Source: CAD feature listing. Evaluate the final solid. Frame: model axes, mm. A direction names the side the tool comes from. Coordinates: 2 decimals unless noted, no trailing zeros. Write each loop counter-clockwise with the first axis right and the second up, starting at its lowest first coordinate (ties: lowest second). Pieces come first, ordered by that corner, then holes. Notation, with made-up numbers: (53.5, -11.75) - (87.5, -11.75) arc R16 ccw to (87.5, 16.25) - close; hole circle Ø6 at (82.25, -23.75). An arc over 180 degrees is marked (long way). One line per question, with ' | ' between items. Start each with the question number.
Q1. Access query for faces 5 (the face through (-116, 4, 58)), 6 (the face through (-121, 3.5, -71)), 7 (the face through (116, 4, 58)), 8 (the face through (104.9, 3.8, -65)). Directions: +Z, -Z, +X, -X, +Y, -Y. A direction counts if a zero-diameter tool reaches every point of the face in a straight line with its end or side. Return the directions, or none.
Q2. Contact query for flat-ended pins moving along their axis: P1, Ø5, axis at x = 60.16, z = -71, coming from the +Y side; P2, Ø1, axis at y = 4.5, z = 50.5, coming from the +X side; P3, Ø1.7, axis at x = -120.5, z = -70, coming from the -Y side; P4, Ø3, axis at x = -122.5, z = 5, coming from the +Y side. Output: stop coordinate, or through.
Q3. Cut plane A-A, the plane z = -3. Return loops of the section in (x, y).
Q4. Line query: line 1 (X direction, y = 3.15, z = 60); line 2 (Z direction, x = 3.5, y = 3.6); line 3 (X direction, y = 3.7, z = -16). Output: solid intervals per line, ascending.
Q5. Draft query along Z for faces 1 (the face through (1, 5, -1)), 2 (the face through (119, 3.5, 69)), 3 (the face through (-121, 3.5, 69)), 4 (the face through (2, 2, 75)). Return one class per face: +Z half, -Z half, draft (parallel to the pull), parting line (faces both ways), or undercut.
```python
from build123d import *

# Parameters (mm, degrees)
EXTRUDE_1_DEPTH     = 5
CUT_EXTRUDE_1_DEPTH = 1.5
CUT_EXTRUDE_2_DEPTH = 2.5
SKETCH_4_R          = 1.25
CUT_EXTRUDE_3_DEPTH = 5
SKETCH_5_R          = 2.85
CUT_EXTRUDE_4_DEPTH = 3.5
SKETCH_6_R          = 1.25
CUT_EXTRUDE_5_DEPTH = 5
SKETCH_7_R          = 2.85
CUT_EXTRUDE_6_DEPTH = 3.5


with BuildPart() as part:
    # 草图1 → 凸台-拉伸1 (new body)
    with BuildSketch(Plane(origin=(0, 0, 0), x_dir=(1, 0, 0), z_dir=(0, 1, 0))):
        with BuildLine():
            Line((-120, 75), (120, 75))
            ThreePointArc((120, 75), (123.535533906, 73.535533906), (125, 70))
            Line((125, 70), (125, -70))
            ThreePointArc((125, -70), (123.535533906, -73.535533906), (120, -75))
            Line((120, -75), (-120, -75))
            ThreePointArc((-120, -75), (-123.535533906, -73.535533906), (-125, -70))
            Line((-125, -70), (-125, 70))
            ThreePointArc((-125, 70), (-123.535533906, 73.535533906), (-120, 75))
        make_face()
    extrude(amount=EXTRUDE_1_DEPTH)

    # 草图2 → 切除-拉伸1 (cut)
    with BuildSketch(Plane(origin=(0, 5, 0), x_dir=(1, 0, 0), z_dir=(0, 1, 0))):
        with BuildLine():
            Line((-125, 60), (-120, 60))
            ThreePointArc((-120, 60), (-116.464466094, 58.535533906), (-115, 55))
            Line((-115, 55), (-115, -55))
            ThreePointArc((-115, -55), (-116.464466094, -58.535533906), (-120, -60))
            Line((-120, -60), (-125, -60))
            Line((-125, -60), (-125, 60))
        make_face()
        with BuildLine():
            Line((115, 55), (115, -55))
            ThreePointArc((115, -55), (116.464466094, -58.535533906), (120, -60))
            Line((120, -60), (125, -60))
            Line((125, -60), (125, 60))
            Line((125, 60), (120, 60))
            ThreePointArc((120, 60), (116.464466094, 58.535533906), (115, 55))
        make_face()
    extrude(amount=-CUT_EXTRUDE_1_DEPTH, mode=Mode.SUBTRACT)

    # 草图3 → 切除-拉伸2 (cut)
    with BuildSketch(Plane(origin=(0, 5, 0), x_dir=(1, 0, 0), z_dir=(0, 1, 0))):
        with BuildLine():
            Line((-100, 67), (100, 67))
            ThreePointArc((100, 67), (104.949747468, 64.949747468), (107, 60))
            Line((107, 60), (107, -60))
            ThreePointArc((107, -60), (104.949747468, -64.949747468), (100, -67))
            Line((100, -67), (-100, -67))
            ThreePointArc((-100, -67), (-104.949747468, -64.949747468), (-107, -60))
            Line((-107, -60), (-107, 60))
            ThreePointArc((-107, 60), (-104.949747468, 64.949747468), (-100, 67))
        make_face()
        with BuildLine():
            Line((-100, 65), (100, 65))
            ThreePointArc((100, 65), (103.535533906, 63.535533906), (105, 60))
            Line((105, 60), (105, -60))
            ThreePointArc((105, -60), (103.535533906, -63.535533906), (100, -65))
            Line((100, -65), (-100, -65))
            ThreePointArc((-100, -65), (-103.535533906, -63.535533906), (-105, -60))
            Line((-105, -60), (-105, 60))
            ThreePointArc((-105, 60), (-103.535533906, 63.535533906), (-100, 65))
        make_face(mode=Mode.SUBTRACT)
    extrude(amount=-CUT_EXTRUDE_2_DEPTH, mode=Mode.SUBTRACT)

    # 草图4 → 切除-拉伸3 (cut)
    with BuildSketch(Plane.XZ):
        with Locations(Location((-120, 70, 0), (0, 0, 270))):
            Circle(SKETCH_4_R)
        with Locations(Location((-120, -70, 0), (0, 0, 270))):
            Circle(SKETCH_4_R)
        with Locations(Location((120, -70, 0), (0, 0, 270))):
            Circle(SKETCH_4_R)
        with Locations(Location((120, 70, 0), (0, 0, 270))):
            Circle(SKETCH_4_R)
    extrude(amount=-CUT_EXTRUDE_3_DEPTH, mode=Mode.SUBTRACT)

    # 草图5 → 切除-拉伸4 (cut)
    with BuildSketch(Plane.XZ):
        with Locations(Location((-120, 70, 0), (0, 0, 270))):
            Circle(SKETCH_5_R)
        with Locations(Location((-120, -70, 0), (0, 0, 270))):
            Circle(SKETCH_5_R)
        with Locations(Location((120, -70, 0), (0, 0, 270))):
            Circle(SKETCH_5_R)
        with Locations(Location((120, 70, 0), (0, 0, 270))):
            Circle(SKETCH_5_R)
    extrude(amount=-CUT_EXTRUDE_4_DEPTH, mode=Mode.SUBTRACT)

    # 草图6 → 切除-拉伸5 (cut)
    with BuildSketch(Plane(origin=(0, 5, 0), x_dir=(1, 0, 0), z_dir=(0, 1, 0))):
        with Locations(Location((0, 71, 0), (0, 0, 270))):
            Circle(SKETCH_6_R)
        with Locations(Location((-60.164669271, 71, 0), (0, 0, 270))):
            Circle(SKETCH_6_R)
        with Locations(Location((60.164669271, 71, 0), (0, 0, 90))):
            Circle(SKETCH_6_R)
        with Locations(Location((60.164669271, -71, 0), (0, 0, 270))):
            Circle(SKETCH_6_R)
        with Locations(Location((-60.164669271, -71, 0), (0, 0, 90))):
            Circle(SKETCH_6_R)
        with Locations(Location((0, -71, 0), (0, 0, 90))):
            Circle(SKETCH_6_R)
    extrude(amount=-CUT_EXTRUDE_5_DEPTH, mode=Mode.SUBTRACT)

    # 草图7 → 切除-拉伸6 (cut)
    with BuildSketch(Plane.XZ):
        with Locations(Location((-60.164669271, 71, 0), (0, 0, 270))):
            Circle(SKETCH_7_R)
        with Locations(Location((0, 71, 0), (0, 0, 270))):
            Circle(SKETCH_7_R)
        with Locations(Location((60.164669271, 71, 0), (0, 0, 270))):
            Circle(SKETCH_7_R)
        with Locations(Location((60.164669271, -71, 0), (0, 0, 90))):
            Circle(SKETCH_7_R)
        with Locations(Location((0, -71, 0), (0, 0, 90))):
            Circle(SKETCH_7_R)
        with Locations(Location((-60.164669271, -71, 0), (0, 0, 90))):
            Circle(SKETCH_7_R)
    extrude(amount=-CUT_EXTRUDE_6_DEPTH, mode=Mode.SUBTRACT)


solid = part.part
```
Reply:
1) face 5: -X, +Y | face 6: -Y | face 7: +X, +Y | face 8: +Y
2) P1: stops at y = 5 | P2: stops at x = 115 | P3: stops at y = 3.5 | P4: stops at y = 3.5
3) outline: (-125, 0) - (125, 0) - (125, 3.5) - (115, 3.5) - (115, 5) - (107, 5) - (107, 2.5) - (105, 2.5) - (105, 5) - (-105, 5) - (-105, 2.5) - (-107, 2.5) - (-107, 5) - (-115, 5) - (-115, 3.5) - (-125, 3.5) - close
4) line 1: x = -125 to -107, -105 to 105, 107 to 125 | line 2: z = -75 to -67, -65 to 65, 67 to 75 | line 3: x = -115 to -107, -105 to 105, 107 to 115
5) face 1: draft | face 2: undercut | face 3: undercut | face 4: +Z half
